from build123d import *

# Parameters (mm, degrees)
F0_W     = 64.7669136524
F0_H     = 30.8674070984
F0_R     = 11
F1_DEPTH = 100
F4_W     = 64.7669136524
F4_H     = 78.3874105722
F6_R     = 11
F7_DEPTH = 75


# Not quite as in the source:
# - the arcs of a loft's sections are written as splines that run evenly, so that the points pair up as in the source's solid


with BuildPart() as f1:
    # F0 (on Top) → F1 (new body, symmetric)
    with BuildSketch(Plane.XY):
        Rectangle(F0_W, F0_H)
        Circle(F0_R, mode=Mode.SUBTRACT)
    extrude(amount=F1_DEPTH, both=True)

    # F4 (on face) → F5 section 0
    with BuildSketch(Plane.XZ.offset(15.4337035492)):
        Rectangle(F4_W, F4_H)
    # F3 (on offset) → F5 section 1
    with BuildSketch(Plane.XZ.offset(90)):
        with BuildLine():
            add(Edge.make_bspline(
                [(13.3759952004, 16.1889700845), (12.3164295861, 17.0644269232), (11.1706673311, 17.8355065906), (8.7506683017, 19.1393549588), (7.4764913666, 19.6720914194), (4.8486237419, 20.4787683169), (3.4949980316, 20.7526888071), (0.7602492908, 21.0311940931), (-0.6208061176, 21.0357720023), (-3.3573411141, 20.7754028748), (-4.7127530359, 20.5104622764), (-7.3459107829, 19.721224575), (-8.623591498, 19.1969469876), (-11.0521812199, 17.9091706745), (-12.203030175, 17.1457037918), (-14.3337225308, 15.4088773887), (-15.3135132459, 14.4355608147), (-16.1889700845, 13.3759952004)],
                knots=[0, 0, 0, 0, 0.125, 0.125, 0.25, 0.25, 0.375, 0.375, 0.5, 0.5, 0.625, 0.625, 0.75, 0.75, 0.875, 0.875, 1, 1, 1, 1], degree=3))
            add(Edge.make_bspline(
                [(-16.1889700845, 13.3759952004), (-17.0644269232, 12.3164295861), (-17.8355065906, 11.1706673311), (-19.1393549588, 8.7506683017), (-19.6720914194, 7.4764913666), (-20.4787683169, 4.8486237419), (-20.7526888071, 3.4949980316), (-21.0311940931, 0.7602492908), (-21.0357720023, -0.6208061176), (-20.7754028748, -3.3573411141), (-20.5104622764, -4.7127530359), (-19.721224575, -7.3459107829), (-19.1969469876, -8.623591498), (-17.9091706745, -11.0521812199), (-17.1457037918, -12.203030175), (-15.4088773887, -14.3337225308), (-14.4355608147, -15.3135132459), (-13.3759952004, -16.1889700845)],
                knots=[0, 0, 0, 0, 0.125, 0.125, 0.25, 0.25, 0.375, 0.375, 0.5, 0.5, 0.625, 0.625, 0.75, 0.75, 0.875, 0.875, 1, 1, 1, 1], degree=3))
            add(Edge.make_bspline(
                [(-13.3759952004, -16.1889700845), (-12.3164295861, -17.0644269232), (-11.1706673311, -17.8355065906), (-8.7506683017, -19.1393549588), (-7.4764913666, -19.6720914194), (-4.8486237419, -20.4787683169), (-3.4949980316, -20.7526888071), (-0.7602492908, -21.0311940931), (0.6208061176, -21.0357720023), (3.3573411141, -20.7754028748), (4.7127530359, -20.5104622764), (7.3459107829, -19.721224575), (8.623591498, -19.1969469876), (11.0521812199, -17.9091706745), (12.203030175, -17.1457037918), (14.3337225308, -15.4088773887), (15.3135132459, -14.4355608147), (16.1889700845, -13.3759952004)],
                knots=[0, 0, 0, 0, 0.125, 0.125, 0.25, 0.25, 0.375, 0.375, 0.5, 0.5, 0.625, 0.625, 0.75, 0.75, 0.875, 0.875, 1, 1, 1, 1], degree=3))
            add(Edge.make_bspline(
                [(16.1889700845, -13.3759952004), (17.0644269232, -12.3164295861), (17.8355065906, -11.1706673311), (19.1393549588, -8.7506683017), (19.6720914194, -7.4764913666), (20.4787683169, -4.8486237419), (20.7526888071, -3.4949980316), (21.0311940931, -0.7602492908), (21.0357720023, 0.6208061176), (20.7754028748, 3.3573411141), (20.5104622764, 4.7127530359), (19.721224575, 7.3459107829), (19.1969469876, 8.623591498), (17.9091706745, 11.0521812199), (17.1457037918, 12.203030175), (15.4088773887, 14.3337225308), (14.4355608147, 15.3135132459), (13.3759952004, 16.1889700845)],
                knots=[0, 0, 0, 0, 0.125, 0.125, 0.25, 0.25, 0.375, 0.375, 0.5, 0.5, 0.625, 0.625, 0.75, 0.75, 0.875, 0.875, 1, 1, 1, 1], degree=3))
        make_face()
    loft(ruled=True)

    # F6 (on face) → F7 (cut)
    with BuildSketch(Plane.XZ.offset(90)):
        Circle(F6_R)
    extrude(amount=-F7_DEPTH, mode=Mode.SUBTRACT)


solid = f1.part
The model under review builds one solid part; all positions refer to its coordinate system, in mm. A direction names the side the tool comes from. Round coordinates to 2 decimals unless told otherwise and drop trailing zeros. Write each loop counter-clockwise with the first axis right and the second up, starting at its lowest first coordinate (ties: lowest second). Pieces come first, ordered by that corner, then holes. Notation, with made-up numbers: (64.25, 87) -> (118.25, 87) arc R19 ccw to (118.25, 101) -> close; hole circle Ø6 at (-1.5, 34.25). An arc over 180 degrees is marked (long way). Answer as a JSON object with one key per item and string values.
1. We need section B-B on z = 76. State the section outline as (x, y) points, and give its area (3 significant figures).
Results found:
{"outline": "(-32.38, -15.43) -> (32.38, -15.43) -> (32.38, 15.43) -> (-32.38, 15.43) -> close; hole circle Ø22 at (0, 0)", "area": "1,620 mm^2"}
2. The part is to be moulded in two halves that separate along Z. For faces 1 (the face through (-8, 11, -100)), 2 (the face through (-2.38, -53.02, -10.74)), 3 (the face through (0, -15.434, 70)), 4 (the face through (0, -15, 0)), say which applies: pulls with the +Z half, pulls with the -Z half, needs draft (parallel to the pull), parting line crosses it, or undercut.
Results found:
{"face 1": "pulls with the -Z half", "face 2": "undercut", "face 3": "needs draft", "face 4": "undercut"}
3. To check wall thickness, follow line 1 along X through (y, z) = (-1, -50.5); line 2 along Y through (x, z) = (0, 48); line 3 along Y through (x, z) = (-20, -64). State the ranges of each line that lie inside material, in increasing order.
Results found:
{"line 1": "x = -32.38 to -10.95, 10.95 to 32.38", "line 2": "y = -15.43 to -11, 11 to 15.43", "line 3": "y = -15.43 to 15.43"}
4. Machinability: for faces 5 (the face through (13, -90, 1)), 6 (the face through (0, -15.434, -69)), which of the approach directions +Z, -Z, +X, -X, +Y, -Y give a long, thin tool a straight path to every point of the face, cutting with its end or side? Answer none if there is none.
Results found:
{"face 5": "+Z, -Z, +X, -X, -Y", "face 6": "-Z, +X, -X, -Y"}
5. Clearance check with flat-ended pins moving along their axes: pin 1 (4 mm diameter, centred on y = -35.5, z = -0.5, fed in from +X); pin 2 (10 mm diameter, centred on x = -15, y = -72, fed in from -Z); pin 3 (1.5 mm diameter, centred on x = 12, y = -63.5, fed in from +Z). State where each tip first meets the part, or that it passes through.
Results found:
{"pin 1": "stops at x = 29.61", "pin 2": "stops at z = -25.15", "pin 3": "stops at z = 26.75"}
6. We need section A-A on y = 0. State the section outline as (x, z) points, and give its area (3 significant figures).
Results found:
{"outline": "(-32.38, -100) -> (-11, -100) -> (-11, 100) -> (-32.38, 100) -> close; (11, -100) -> (32.38, -100) -> (32.38, 100) -> (11, 100) -> close", "area": "8,550 mm^2"}
